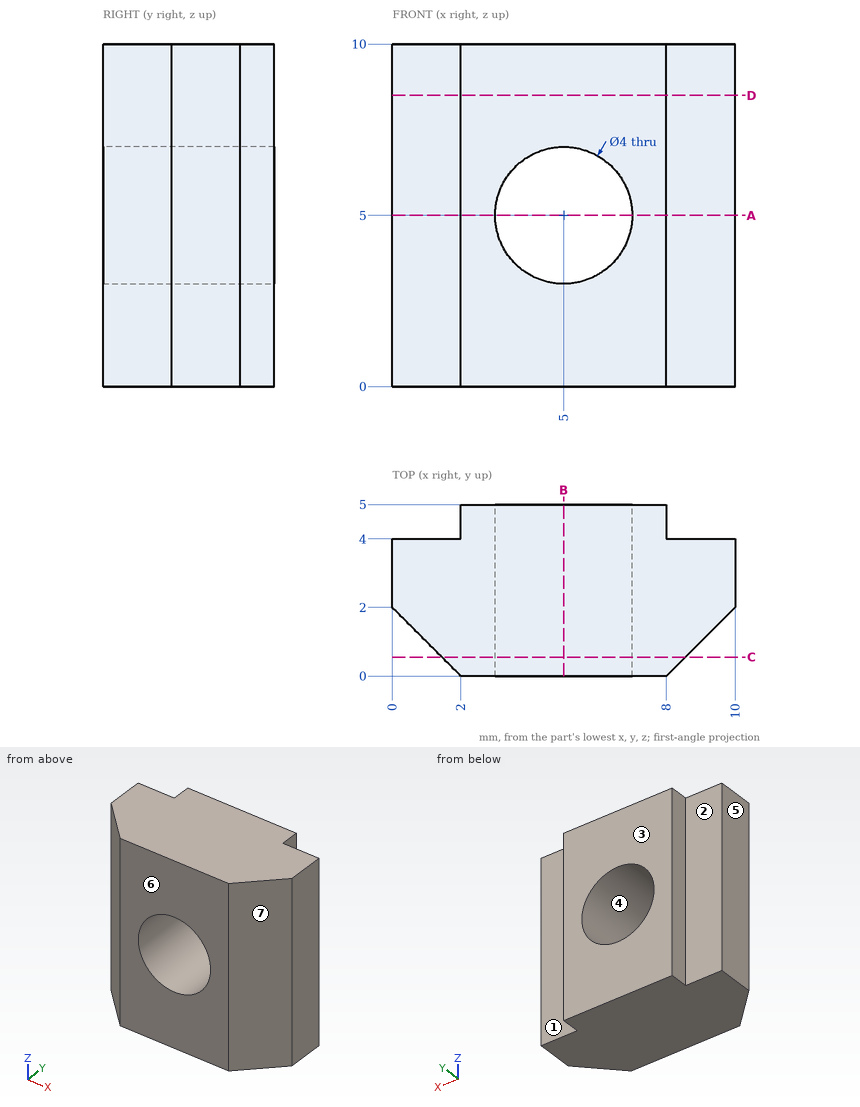
The figure shows three views and two pictorial views of one solid part (mm, origin at its lowest corner). Answer the questions. A direction names the side the tool comes from. Coordinates: 2 decimals unless noted, no trailing zeros. Loops run counter-clockwise (first coordinate to the right, second up) from the corner with the lowest first, then second, coordinate; pieces in that order, holes last. Notation, with made-up numbers: (11.25, 39.5) -> (51.25, 39.5) arc R19 ccw to (51.25, 63.5) -> close; hole circle Ø7 at (3, 16). An arc over 180 degrees is marked (long way). Write item = value, one per line. Start each with the question number.
1) A cutting plane is placed at A-A (z = 5). Give the vertices of the cut face in (x, y).
2) Given pin 1 Ø0.8 at (y, z) = (4.5, 4) entering from +X; pin 2 Ø6 at (x, z) = (3.5, 7) entering from -Y; pin 3 Ø1 at (x, z) = (0.5, 5.5) entering from +Y, each flat-ended and moving along its own axis, determine where each tip first touches the part or whether it passes through.
3) A cutting plane is placed at C-C (y = 0.55). Give the vertices of the cut face in (x, z), then the cut area to 3 significant figures.
4) The mould has two halves that part along X. Classify the marked faces 4, 5, 6 and 7: released by +X, released by -X, zero draft, split by the parting line, or undercut.
5) Straight lines are drawn through the part: line 1 (X direction, y = 2.15, z = 5); line 2 (Z direction, x = 6.75, y = 0.65); line 3 (X direction, y = 4.05, z = 1.5). For each, find the intervals that lie inside material, in ascending order. Write a range as from..to.
6) A tool of negligible diameter and unlimited length cuts with its end or side. For the marked faces 1, 2 and 3, from which of +Z, -Z, +X, -X, +Y, -Y can it reach the whole face along a straight path? Write none if from no direction.
7) A cutting plane is placed at B-B (x = 5). Give the vertices of the cut face in (y, z).
8) A cutting plane is placed at D-D (z = 8.5). Give the vertices of the cut face in (x, y), then the cut area to 3 significant figures.
Responses:
q1.outline = (0, 2) -> (2, 0) -> (3, 0) -> (3, 5) -> (2, 5) -> (2, 4) -> (0, 4) -> close; (7, 0) -> (8, 0) -> (10, 2) -> (10, 4) -> (8, 4) -> (8, 5) -> (7, 5) -> close
q2.pin_1 = 8
q2.pin_2 = 0
q2.pin_3 = 4
q3.outline = (1.45, 0) -> (8.55, 0) -> (8.55, 10) -> (1.45, 10) -> close; hole circle Ø4 at (5, 5)
q3.area = 58.4 mm²
q4.face_4 = undercut
q4.face_5 = released by -X
q4.face_6 = zero draft
q4.face_7 = released by +X
q5.line_1 = 0..3, 7..10
q5.line_2 = 0..4.03, 5.97..10
q5.line_3 = 2..8
q6.face_1 = +Z, -Z, +X, +Y
q6.face_2 = +Z, -Z, -X, +Y
q6.face_3 = +Z, -Z, +X, -X, +Y
q7.outline = (0, 0) -> (5, 0) -> (5, 3) -> (0, 3) -> close; (0, 7) -> (5, 7) -> (5, 10) -> (0, 10) -> close
q8.outline = (0, 2) -> (2, 0) -> (8, 0) -> (10, 2) -> (10, 4) -> (8, 4) -> (8, 5) -> (2, 5) -> (2, 4) -> (0, 4) -> close
q8.area = 42.0 mm²
